Design review of the part built by this model. Coordinates are the model's own, in mm. Round coordinates to 2 decimals unless told otherwise and drop trailing zeros. Order: outer loops, then holes, each group sorted by start corner. A loop starts at its lowest first (then second) coordinate and runs counter-clockwise, first axis right, second up. Notation, with made-up numbers: M 32,-3.75 L 87,-3.75 A11 ccw 87,7.25 Z; hole C 34.25,-15.5 d4. An arc over 180 degrees is marked long. Use a Markdown table: item, result. Add a question column.
(1) Take a section at C-C (x = 25.8). Write out the cut boundary in (y, z), then the cut area to 3 significant figures.
(2) Take a section at D-D (x = 11.5). Write out the cut boundary in (y, z).
(3) Take a section at B-B (y = -47.5). Write out the cut boundary in (x, z).
(4) For pin 1 (2.5 mm diameter, centred on x = -11.46, y = -69.72, fed in from +Z), flat-tipped, find the tip position at first contact; note if it passes through.
(5) Take a section at A-A (x = -15.5). Write out the cut boundary in (y, z).
(6) To check wall thickness, follow probe 1 along Y at (x, z) = (14, 0.4); probe 2 along X at (y, z) = (-64.5, 1.3); probe 3 along X at (y, z) = (-67.5, 1.8). State the ranges of each line that lie inside material, in increasing order. Write a range as from..to.
```python
from build123d import *
from build123d.topology import SkipClean

# Parameters (mm, degrees)
SKETCH1_R           = 1.5
SKETCH1_R_2         = 1.25
BOSS_EXTRUDE1_DEPTH = 2
SKETCH2_W           = 50.695336344
SKETCH2_H           = 10.606019708
CUT_EXTRUDE1_DEPTH  = 40.656761755
CUT_EXTRUDE2_START  = -26.91026
SKETCH2_2_W         = 50.695336344
SKETCH2_2_H         = 10.606019708
CUT_EXTRUDE2_DEPTH  = 13.746501755
FILLET1_R           = 2


with BuildPart() as part:
    # Sketch1 → Boss-Extrude1 (new body)
    with BuildSketch(Plane.XY):
        with BuildLine():
            ThreePointArc((13.788582233, -49.138227177), (13.939896438, -48.976395169), (14.080010805, -48.804774799))
            Line((14.080010805, -48.804774799), (22.226347675, -48.804774799))
            Line((22.226347675, -48.804774799), (24.385786438, -50.964213562))
            ThreePointArc((24.385786438, -50.964213562), (27.214213562, -50.964213562), (27.214213562, -48.135786438))
            Line((27.214213562, -48.135786438), (24.468988362, -45.390561237))
            ThreePointArc((24.468988362, -45.390561237), (23.820141664, -44.957015734), (23.054774799, -44.804774799))
            Line((23.054774799, -44.804774799), (14.080010805, -44.804774799))
            ThreePointArc((14.080010805, -44.804774799), (11.676557666, -43.51221201), (9.121677477, -44.471322421))
            Line((9.121677477, -44.471322421), (5.27936576, -48.313634139))
            ThreePointArc((5.27936576, -48.313634139), (4.318629382, -48.847331879), (3.220960165, -48.792834589))
            ThreePointArc((3.220960165, -48.792834589), (0, -48.259904655), (-3.220960165, -48.792834589))
            ThreePointArc((-3.220960165, -48.792834589), (-4.318629382, -48.847331879), (-5.27936576, -48.313634139))
            Line((-5.27936576, -48.313634139), (-9.121677477, -44.471322421))
            ThreePointArc((-9.121677477, -44.471322421), (-11.676557666, -43.51221201), (-14.080010805, -44.804774799))
            Line((-14.080010805, -44.804774799), (-23.054774799, -44.804774799))
            ThreePointArc((-23.054774799, -44.804774799), (-23.820141664, -44.957015734), (-24.468988362, -45.390561237))
            Line((-24.468988362, -45.390561237), (-27.214213562, -48.135786438))
            ThreePointArc((-27.214213562, -48.135786438), (-27.214213562, -50.964213562), (-24.385786438, -50.964213562))
            Line((-24.385786438, -50.964213562), (-22.226347675, -48.804774799))
            Line((-22.226347675, -48.804774799), (-14.080010805, -48.804774799))
            ThreePointArc((-14.080010805, -48.804774799), (-13.939896438, -48.976395169), (-13.788582233, -49.138227177))
            Line((-13.788582233, -49.138227177), (-9.946270516, -52.980538895))
            ThreePointArc((-9.946270516, -52.980538895), (-9.412572775, -53.941275272), (-9.467070065, -55.03894449))
            ThreePointArc((-9.467070065, -55.03894449), (-10, -58.259904655), (-9.467070065, -61.480864819))
            ThreePointArc((-9.467070065, -61.480864819), (-9.412572775, -62.578534037), (-9.946270516, -63.539270415))
            Line((-9.946270516, -63.539270415), (-13.788582233, -67.381582132))
            ThreePointArc((-13.788582233, -67.381582132), (-13.939896438, -67.54341414), (-14.080010805, -67.71503451))
            Line((-14.080010805, -67.71503451), (-21.456538365, -67.71503451))
            Line((-21.456538365, -67.71503451), (-24.385786438, -64.785786438))
            ThreePointArc((-24.385786438, -64.785786438), (-27.214213562, -64.785786438), (-27.214213562, -67.614213562))
            Line((-27.214213562, -67.614213562), (-23.699179053, -71.129248072))
            ThreePointArc((-23.699179053, -71.129248072), (-23.050332355, -71.562793575), (-22.28496549, -71.71503451))
            Line((-22.28496549, -71.71503451), (-14.080010805, -71.71503451))
            ThreePointArc((-14.080010805, -71.71503451), (-11.676557666, -73.0075973), (-9.121677477, -72.048486888))
            Line((-9.121677477, -72.048486888), (-5.27936576, -68.20617517))
            ThreePointArc((-5.27936576, -68.20617517), (-4.318629382, -67.67247743), (-3.220960165, -67.72697472))
            ThreePointArc((-3.220960165, -67.72697472), (0, -68.259904655), (3.220960165, -67.72697472))
            ThreePointArc((3.220960165, -67.72697472), (4.318629382, -67.67247743), (5.27936576, -68.20617517))
            Line((5.27936576, -68.20617517), (9.121677477, -72.048486888))
            ThreePointArc((9.121677477, -72.048486888), (11.676557666, -73.0075973), (14.080010805, -71.71503451))
            Line((14.080010805, -71.71503451), (22.28496549, -71.71503451))
            ThreePointArc((22.28496549, -71.71503451), (23.050332355, -71.562793575), (23.699179053, -71.129248072))
            Line((23.699179053, -71.129248072), (27.214213562, -67.614213562))
            ThreePointArc((27.214213562, -67.614213562), (27.214213562, -64.785786438), (24.385786438, -64.785786438))
            Line((24.385786438, -64.785786438), (21.456538365, -67.71503451))
            Line((21.456538365, -67.71503451), (14.080010805, -67.71503451))
            ThreePointArc((14.080010805, -67.71503451), (13.939896438, -67.54341414), (13.788582233, -67.381582132))
            Line((13.788582233, -67.381582132), (9.946270516, -63.539270415))
            ThreePointArc((9.946270516, -63.539270415), (9.412572775, -62.578534037), (9.467070065, -61.480864819))
            ThreePointArc((9.467070065, -61.480864819), (10, -58.259904655), (9.467070065, -55.03894449))
            ThreePointArc((9.467070065, -55.03894449), (9.412572775, -53.941275272), (9.946270516, -52.980538895))
            Line((9.946270516, -52.980538895), (13.788582233, -49.138227177))
        make_face()
        with Locations((-7.820715031, -50.439189624)):
            Circle(SKETCH1_R, mode=Mode.SUBTRACT)
        with Locations((7.820715031, -50.439189624)):
            Circle(SKETCH1_R, mode=Mode.SUBTRACT)
        with Locations((25.8, -49.55)):
            Circle(SKETCH1_R_2, mode=Mode.SUBTRACT)
        with Locations((11.455129855, -69.71503451)):
            Circle(SKETCH1_R, mode=Mode.SUBTRACT)
        with Locations((-25.8, -49.55)):
            Circle(SKETCH1_R_2, mode=Mode.SUBTRACT)
        with Locations((25.8, -66.2)):
            Circle(SKETCH1_R_2, mode=Mode.SUBTRACT)
        with Locations((-11.455129855, -69.71503451)):
            Circle(SKETCH1_R, mode=Mode.SUBTRACT)
        with Locations((-25.8, -66.2)):
            Circle(SKETCH1_R_2, mode=Mode.SUBTRACT)
    extrude(amount=BOSS_EXTRUDE1_DEPTH)

    # Sketch2 → Cut-Extrude1 (cut, through all)
    with BuildSketch(Plane(origin=(0, -44.804774799, 0), x_dir=(1, 0, 0), z_dir=(0, 1, 0))):
        Rectangle(SKETCH2_W, SKETCH2_H)
    extrude(amount=CUT_EXTRUDE1_DEPTH, mode=Mode.SUBTRACT)

    # Sketch2<2> → Cut-Extrude2 (cut, through all)
    with SkipClean():  # the faces are left unmerged after this step: merging them gives an invalid solid
        with BuildSketch(Plane(origin=(0, -44.804774799, 0), x_dir=(1, 0, 0), z_dir=(0, 1, 0)).offset(CUT_EXTRUDE2_START)):
            Rectangle(SKETCH2_2_W, SKETCH2_2_H)
        extrude(amount=-CUT_EXTRUDE2_DEPTH, mode=Mode.SUBTRACT)

    # Fillet1
    fillet1_edges = [part.edges().sort_by_distance(p)[0] for p in [
        (-8.788225099, -44.804774799, 1),
        (8.788225099, -44.804774799, 1),
        (8.788225389, -71.715034799, 1),
        (-8.788225389, -71.715034799, 1),
    ]]
    fillet(fillet1_edges, radius=FILLET1_R)


solid = part.part
```
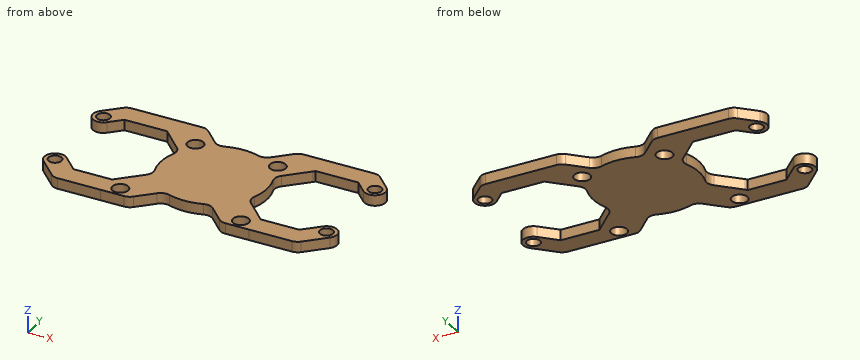
Verdict:
| question | item | result |
|---|---|---|
| 1 | outline | M -69.03,0 L -67.45,0 L -67.45,2 L -69.03,2 Z; M -64.95,0 L -64.2,0 L -64.2,2 L -64.95,2 Z; M -51.55,0 L -50.8,0 L -50.8,2 L -51.55,2 Z; M -48.3,0 L -46.72,0 L -46.72,2 L -48.3,2 Z |
| 1 | area | 9.31 mm^2 |
| 2 | outline | M -71.72,0 L -71.21,0 L -71.21,2 L -71.72,2 Z; M -68.22,0 L -65.09,0 L -65.09,2 L -68.22,2 Z; M -51.43,0 L -44.8,0 L -44.8,2 L -51.43,2 Z |
| 3 | outline | M -26.58,0 L -6.09,0 L -6.09,2 L -26.58,2 Z; M 6.09,0 L 26.58,0 L 26.58,2 L 6.09,2 Z |
| 4 | pin 1 | passes through |
| 5 | outline | M -71.72,0 L -67.72,0 L -67.72,2 L -71.72,2 Z; M -48.8,0 L -44.8,0 L -44.8,2 L -48.8,2 Z |
| 6 | probe 1 | y = -71.72..-67.61, -48.91..-44.8 |
| 6 | probe 2 | x = -26.85..-24.75, -10.91..10.91, 24.75..26.85 |
| 6 | probe 3 | x = -27.32..-21.67, -13.9..13.9, 21.67..27.32 |
